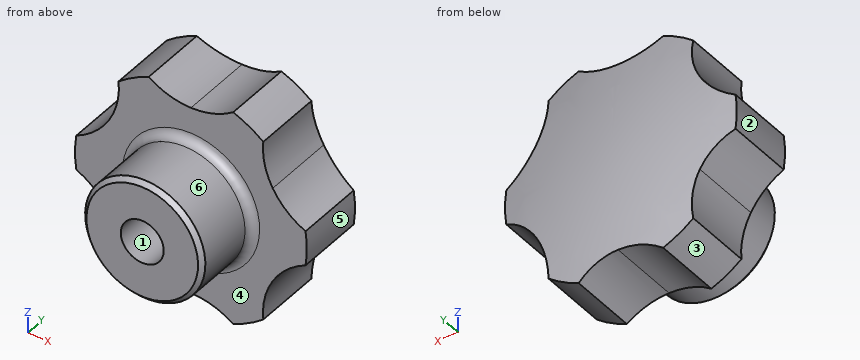
```python
from build123d import *

# Parameters (mm, degrees)
CHAMFER_1_SIZE           = 1
CUT_EXTRUDE_1_DEPTH      = 43.576377572
PATTERN_CIRCULAR_1_COUNT = 6
MM_1_D                   = 10
MM_1_DEPTH               = 20
MM_1_TIP                 = 3.004303095


with BuildPart() as part:
    # 草图1 → 旋转1 (revolve)
    with BuildSketch(Plane.XY, mode=Mode.PRIVATE) as revolve_1_sk:
        with BuildLine():
            Line((0, 17.5), (0, -17.5))
            Line((0, -17.5), (-14, -17.5))
            Line((-14, -17.5), (-14, -3.334753175))
            ThreePointArc((-14, -3.334753175), (-14.585786438, -1.920539613), (-16, -1.334753175))
            Line((-16, -1.334753175), (-27, -1.334753175))
            Line((-27, -1.334753175), (-27, 14.665246825))
            ThreePointArc((-27, 14.665246825), (-13.574201869, 16.789369415), (0, 17.5))
        make_face()
    revolve(revolve_1_sk.sketch.rotate(Axis((0, 51.094488189, 0), (0, -1, 0)), 270), axis=Axis((0, 51.094488189, 0), (0, -1, 0)))

    # 倒角1
    chamfer_1_edges = [part.edges().sort_by_distance(p)[0] for p in [
        (0, -17.5, -14),
    ]]
    chamfer(chamfer_1_edges, length=CHAMFER_1_SIZE)

    # 草图3 → 切除-拉伸1 (cut, through all)
    with BuildSketch(Plane.XZ.offset(1.334753175)):
        with BuildLine():
            ThreePointArc((9.845244015, 25.141025641), (5.009606157, 26.531186294), (0, 27))
            Line((0, 27), (0, 22))
            ThreePointArc((-2.3e-08, 22), (5.167080204, 22.804281981), (9.845244015, 25.141025641))
        make_face()
        with BuildLine():
            Line((0, 22), (0, 27))
            ThreePointArc((0, 27), (-5.009606157, 26.531186294), (-9.845244015, 25.141025641))
            ThreePointArc((-9.845244015, 25.141025641), (-5.167080226, 22.804281988), (-2.3e-08, 22))
        make_face()
    cut_extrude_1 = extrude(amount=-CUT_EXTRUDE_1_DEPTH, mode=Mode.SUBTRACT)

    # 阵列(圆周)1: 切除-拉伸1 ×6 about axis
    pattern_circular_1_axis = Axis((0, 0, 0), (0, 1, 0))
    for i in range(1, PATTERN_CIRCULAR_1_COUNT):
        add(cut_extrude_1.rotate(pattern_circular_1_axis, i * 360 / PATTERN_CIRCULAR_1_COUNT), mode=Mode.SUBTRACT)

    # 大小mm 暗销孔1
    with Locations(Plane(origin=(0, -17.5, 0), x_dir=(-1, 0, 0), z_dir=(0, -1, 0))):
        with Locations((0, 0)):
            Hole(MM_1_D / 2, depth=MM_1_DEPTH)
            with Locations((0, 0, -(MM_1_DEPTH + MM_1_TIP / 2))):  # 118° drill point
                Cone(0, MM_1_D / 2, MM_1_TIP, mode=Mode.SUBTRACT)


solid = part.part
```
The listing builds one solid part. Answer for the finished solid, in the listing's coordinates (mm). Face numbers are marked on the shaded views. A direction names the side the tool comes from. Give positions to 0.01 mm unless a question says otherwise; leave off trailing zeros. Order: outer loops, then holes, each group sorted by start corner. A loop starts at its lowest first (then second) coordinate and runs counter-clockwise, first axis right, second up.
1) Given P1, Ø4, axis at x = -17, z = -10, coming from the +Y side; P2, Ø6, axis at y = 2.5, z = 8, coming from the -X side; P3, Ø8, axis at x = 0, z = 0, coming from the -Y side, each flat-ended and moving along its own axis, determine where each tip first touches the part or whether it passes through.
Reported:
P1: stops at y = 16.29
P2: stops at x = -24.9
P3: stops at y = 3.1
2) Find section D-D on z = 20. Write down the section's boundary in (x, y).
Reported:
outline: (-16.78, -1.33) - (16.78, -1.33) - (16.78, 14.85) arc R128.45 ccw to (-16.78, 14.85) - close
3) Find section B-B on y = -6.5. Write down the section's boundary in (x, z), then the cut area to 3 significant figures.
Reported:
outline: circle Ø28 at (0, 0); hole circle Ø10 at (0, 0)
area: 537 mm2
4) For the marked faces 5 and 6, determine the directions among +Z, -Z, +X, -X, +Y, -Y from which every point of the face is accessible in a straight line to the end or side of a thin tool.
Reported:
face 5: +X, +Y, -Y
face 6: -Y
5) Consider line 1 along X through (y, z) = (5.5, 20); line 2 along Z through (x, y) = (11, -15); line 3 along Y through (x, z) = (5, -11). Determine where each line is inside the solid, lowest interval first.
Reported:
line 1: x = -16.78 to 16.78
line 2: z = -8.66 to 8.66
line 3: y = -17.5 to 16.94
6) Determine the mould class of the marked faces 1, 2, 3 and 4 for opening direction Z: pulls with the +Z half, pulls with the -Z half, needs draft (parallel to the pull), parting line crosses it, or undercut.
Reported:
face 1: undercut
face 2: parting line crosses it
face 3: pulls with the -Z half
face 4: needs draft
7) Find section A-A on y = 13. Write down the section's boundary in (x, z) (3 decimals), then the cut area to 3 significant figures.
Reported:
outline: (-26.695, -4.044) arc R17 cw to (-16.85, -21.097) arc R27 ccw to (-9.845, -25.141) arc R17 cw to (9.845, -25.141) arc R27 ccw to (16.85, -21.097) arc R17 cw to (26.695, -4.044) arc R27 ccw to (26.695, 4.044) arc R17 cw to (16.85, 21.097) arc R27 ccw to (9.845, 25.141) arc R17 cw to (-9.845, 25.141) arc R27 ccw to (-16.85, 21.097) arc R17 cw to (-26.695, 4.044) arc R27 ccw to start
area: 1,890 mm2
8) Find section C-C on x = -21.5. Write down the section's boundary in (y, z), then the cut area to 3 significant figures.
Reported:
outline: (-1.33, -7.74) - (15.48, -7.74) arc R128.21 ccw to (15.48, 7.74) - (-1.33, 7.74) - close
area: 263 mm2
